from build123d import *

# Parameters (mm, degrees)
SKETCH_1_R               = 15
SKETCH_1_R_2             = 10.25
EXTRUDE_1_DEPTH          = 10
CUT_EXTRUDE_1_DEPTH      = 24.452078799
CUT_EXTRUDE_1_DEPTH_BACK = 24.452078799
SKETCH_2_R               = 3.1
SKETCH_3_R               = 12
SKETCH_3_R_2             = 7
EXTRUDE_2_DEPTH          = 10
EXTRUDE_3_DEPTH          = 10
FILLET_1_R               = 5
CHAMFER_1_SIZE           = 1


with BuildPart() as part:
    # Sketch 1 → Extrude 1 (new, symmetric)
    with BuildSketch(Plane.XY):
        Circle(SKETCH_1_R)
        Circle(SKETCH_1_R_2, mode=Mode.SUBTRACT)
    extrude(amount=EXTRUDE_1_DEPTH, both=True)

    # Sketch 2 → Cut-Extrude 1 (cut, two sides: drawn at the far end of the back side and taken through both)
    with BuildSketch(Plane(origin=(0, 0, 0), x_dir=(0, 0, -1), z_dir=(1, 0, 0)).offset(-CUT_EXTRUDE_1_DEPTH_BACK)):
        Circle(SKETCH_2_R)
    extrude(amount=CUT_EXTRUDE_1_DEPTH + CUT_EXTRUDE_1_DEPTH_BACK, mode=Mode.SUBTRACT)



with BuildPart() as body_2:
    # Sketch 3 → Extrude 2 (new, symmetric)
    with BuildSketch(Plane.XY):
        with Locations((50, -10)):
            Circle(SKETCH_3_R)
        with Locations((50, -10)):
            Circle(SKETCH_3_R_2, mode=Mode.SUBTRACT)
    extrude(amount=EXTRUDE_2_DEPTH, both=True)


with BuildPart() as part_1:
    add(part.part)

    add(body_2.part)  # Extrude 3 merges body 2
    # Sketch 4 → Extrude 3 (add, symmetric)
    with BuildSketch(Plane.XY):
        with BuildLine():
            Line((40.202041029, -15), (0, -15))
            ThreePointArc((0, -15), (8.660254038, -12.247448714), (14.142135624, -5))
            Line((14.142135624, -5), (40.202041029, -5))
            ThreePointArc((40.202041029, -5), (39, -10), (40.202041029, -15))
        make_face()
    extrude(amount=EXTRUDE_3_DEPTH, both=True)

    # Fillet 1
    # the kernel refuses this fillet: 5 mm, written as the material it adds along each edge
    with BuildSketch(Plane(origin=(14.142135624, -5, -10), x_dir=(0.1691019787257651, 0.9855985596534883, 0), z_dir=(0, 0, 1))) as fillet_1_piece_1_section:
        with BuildLine():
            CenterArc((5.918569255, -4.927992798), FILLET_1_R, 99.735610317, 90)
            Line((0.990576457, -5.773502692), (0, 0))
            ThreePointArc((0, 0), (2.536529681, -0.216021605), (5.073059362, 0))
        make_face()
    fillet_1_piece_1 = extrude(amount=20, mode=Mode.PRIVATE)
    fillet_1_piece_1 = fillet_1_piece_1 - Plane(origin=(15.878746953, 0, 0), x_dir=(0, 0, -1), z_dir=(-1, 0, 0)) * Cylinder(3.1, 64, mode=Mode.PRIVATE)
    add(fillet_1_piece_1)
    with BuildSketch(Plane(origin=(39.091287885, -15, -10), x_dir=(0.5049509852949774, -0.8631480188528684, 0), z_dir=(0, 0, 1))) as fillet_1_piece_2:
        with BuildLine():
            CenterArc((2.882176688, -4.975245074), FILLET_1_R, 95.70378036, 53.968120928)
            Line((-1.433563406, -2.450490147), (0, 0))
            ThreePointArc((0, 0), (1.192624836, -0.059411824), (2.385249673, 0))
        make_face()
    extrude(amount=20)
    with BuildSketch(Plane(origin=(39.091287885, -5, -10), x_dir=(-1, 0, 0), z_dir=(0, 0, 1))) as fillet_1_piece_3:
        with BuildLine():
            CenterArc((2.83901497, -5), FILLET_1_R, 90, 53.968120928)
            ThreePointArc((-1.204434172, -2.058823529), (-0.550935888, -1.059411824), (0, 0))
            Line((0, 0), (2.83901497, 0))
        make_face()
    extrude(amount=20)

    # Chamfer 1
    chamfer_1_edges = [part_1.edges().sort_by_distance(p)[0] for p in [
        (18.126136458, -15, -10),
        (18.126136458, -15, 10),
        (62, -10, -10),
        (-10.25, 0, -10),
        (62, -10, 10),
        (28.126136458, -5, -10),
        (-10.25, 0, 10),
        (28.126136458, -5, 10),
        (-10.606601718, 10.606601718, -10),
        (-10.606601718, 10.606601718, 10),
        (38.520985948, -15.544336057, -10),
        (38.520985948, -15.544336057, 10),
        (38.520985948, -4.455663943, 10),
        (38.520985948, -4.455663943, -10),
        (16.464466094, -3.535533906, -10),
        (16.464466094, -3.535533906, 10),
    ]]
    chamfer(chamfer_1_edges, length=CHAMFER_1_SIZE)


solid = part_1.part
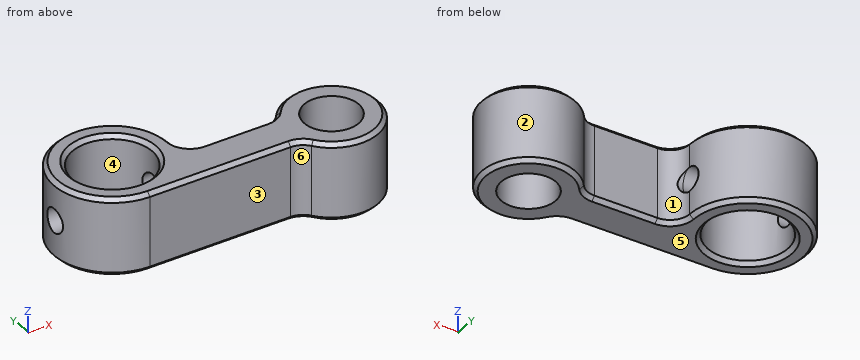
For this review, take the finished solid that the model builds, in its own axes (mm). Face numbers are marked on the shaded views. A direction names the side the tool comes from. Coordinates: 2 decimals unless noted, no trailing zeros. Order: outer loops, then holes, each group sorted by start corner. A loop starts at its lowest first (then second) coordinate and runs counter-clockwise, first axis right, second up. Notation, with made-up numbers: (24, 67.25) -> (66, 67.25) arc R29 ccw to (66, 91.25) -> close; hole circle Ø3 at (-1.75, 14). An arc over 180 degrees is marked (long way). Return JSON: item names as keys, results as strings.
1. We need section C-C on z = 5.5. Write out the cut boundary in (x, y).
Answer block:
{"outline": "(0, -15) -> (36.25, -15) arc R5 cw to (40.3, -17.06) arc R12 ccw (long way) to (40.3, -2.94) arc R5 cw to (36.25, -5) -> (20, -5) arc R5 cw to (15, 0) arc R15 ccw (long way) to start; hole circle Ø20.5 at (0, 0); hole circle Ø14 at (50, -10)"}
2. We need section D-D on y = -2. State how many separate pieces and enclosed holes the cut face has, and give its area (3 significant figures).
Answer block:
{"separate pieces": "5", "enclosed holes": "0", "area": "506 mm²"}
3. For pin 1 Ø1 at (x, z) = (2, 2.5) entering from -Y; pin 2 Ø18 at (x, y) = (50, -10) entering from +Z; pin 3 Ø8 at (x, z) = (-4.5, 6.5) entering from +Y; pin 4 Ø5.5 at (y, z) = (0, 0) entering from +X, all flat-tipped, find the tip position at first contact; note any pin that passes through.
Answer block:
{"pin 1": "y = -15", "pin 2": "z = 10", "pin 3": "y = 14.99", "pin 4": "x = 59.56"}
4. We need section B-B on z = 0. Write out the cut boundary in (x, y).
Answer block:
{"outline": "(-14.68, -3.1) arc R15 ccw to (0, -15) -> (36.25, -15) arc R5 cw to (40.3, -17.06) arc R12 ccw (long way) to (40.3, -2.94) arc R5 cw to (36.25, -5) -> (20, -5) arc R5 cw to (16.08, -3.1) -> (9.77, -3.1) arc R10.25 cw to (-9.77, -3.1) -> close; (-14.68, 3.1) -> (-9.77, 3.1) arc R10.25 cw to (9.77, 3.1) -> (14.68, 3.1) arc R15 ccw to start; hole circle Ø14 at (50, -10)"}
5. For line 1 (Y direction, x = 0, z = 4.5); line 2 (Z direction, x = 11.7, y = 0); line 3 (Y direction, x = 50, z = -1.5), list the stretches that pass through material, from the lowest coordinate up. Write a range as from..to.
Answer block:
{"line 1": "-15..-10.25, 10.25..15", "line 2": "-10..-3.1, 3.1..10", "line 3": "-22..-17, -3..2"}
6. We need section A-A on x = 50. Write out the cut boundary in (y, z).
Answer block:
{"outline": "(-22, -9) -> (-21, -10) -> (-17, -10) -> (-17, 10) -> (-21, 10) -> (-22, 9) -> close; (-3, -10) -> (1, -10) -> (2, -9) -> (2, 9) -> (1, 10) -> (-3, 10) -> close"}
7. Machinability: for the marked faces 1, 2 and 3, which of the approach directions +Z, -Z, +X, -X, +Y, -Y give a long, thin tool a straight path to every point of the face, cutting with its end or side? Answer none if there is none.
Answer block:
{"face 1": "+Z, -Z, +Y", "face 2": "+Z, -Z", "face 3": "+Z, -Z, -X, -Y"}
8. The part is to be moulded in two halves that separate along X. For the marked faces 4, 5 and 6, say which applies: +X half, -X half, draft (parallel to the pull), parting line (faces both ways), or undercut.
Answer block:
{"face 4": "undercut", "face 5": "draft", "face 6": "-X half"}
